from build123d import *

# Parameters (mm, degrees)
F0_R     = 6.35
F1_DEPTH = 2.54
F2_R     = 0.381
F3_DEPTH = 11.938
F4_W     = 0.254
F4_H     = 3.2643415034
F5_DEPTH = 10.7696
F6_R     = 1.524
F7_DEPTH = 2.5654


with BuildPart() as f1:
    # F0 (on Front) → F1 (new body)
    with BuildSketch(Plane.XZ):
        Circle(F0_R)
    extrude(amount=F1_DEPTH)

    # F2 (on Front) → F3 (cut)
    with BuildSketch(Plane.XZ):
        with Locations((0, 2.9252786189)):
            Circle(F2_R)
    extrude(amount=F3_DEPTH, mode=Mode.SUBTRACT)

    # F4 (on Front) → F5 (cut)
    with BuildSketch(Plane.XZ):
        with Locations((-0.0004456008, 4.9322359264)):
            Rectangle(F4_W, F4_H)
    extrude(amount=F5_DEPTH, mode=Mode.SUBTRACT)

    # F6 (on Front) → F7 (join)
    with BuildSketch(Plane.XZ):
        Circle(F6_R)
        with BuildLine():
            add(Edge.make_bspline(
                [(-0.2672408938, -0.7273242873), (-0.3560866168, -0.8291747878), (-0.5301318635, -0.8291747878)],
                knots=[0, 0, 0, 1, 1, 1], degree=2))
            add(Edge.make_bspline(
                [(-0.5301318635, -0.8291747878), (-0.6098620882, -0.8291747878), (-0.6691735969, -0.812402271)],
                knots=[0, 0, 0, 1, 1, 1], degree=2))
            Line((-0.6691735969, -0.812402271), (-0.6691735969, -0.6164798285))
            add(Edge.make_bspline(
                [(-0.6691735969, -0.6164798285), (-0.6084036085, -0.6315507856), (-0.5583291381, -0.6315507856)],
                knots=[0, 0, 0, 1, 1, 1], degree=2))
            add(Edge.make_bspline(
                [(-0.5583291381, -0.6315507856), (-0.4807866329, -0.6315507856), (-0.4473631393, -0.5832994149)],
                knots=[0, 0, 0, 1, 1, 1], degree=2))
            add(Edge.make_bspline(
                [(-0.4473631393, -0.5832994149), (-0.4139396457, -0.5350480441), (-0.4139396457, -0.4324683037)],
                knots=[0, 0, 0, 1, 1, 1], degree=2))
            Line((-0.4139396457, -0.4324683037), (-0.4139396457, 0.6081569771))
            Line((-0.4139396457, 0.6081569771), (-0.1783951708, 0.6081569771))
            Line((-0.1783951708, 0.6081569771), (-0.1783951708, -0.431009824))
            add(Edge.make_bspline(
                [(-0.1783951708, -0.431009824), (-0.1783951708, -0.6254737868), (-0.2672408938, -0.7273242873)],
                knots=[0, 0, 0, 1, 1, 1], degree=2))
        make_face(mode=Mode.SUBTRACT)
        Polygon((0.3328019713, -0.0634729344), (0.3328019713, -0.5024753303), (0.1011467757, -0.5024753303), (0.1011467757, 0.6081569771), (0.7377731738, 0.6081569771), (0.7377731738, 0.415151494), (0.3328019713, 0.415151494), (0.3328019713, 0.1288033088), (0.7095758992, 0.1288033088), (0.7095758992, -0.0634729344), align=None, mode=Mode.SUBTRACT)
    extrude(amount=F7_DEPTH)


solid = f1.part
Could you check a few things on this model? Use its own coordinates, in mm. A direction names the side the tool comes from. Round coordinates to 2 decimals unless told otherwise and drop trailing zeros. Loops run counter-clockwise (first coordinate to the right, second up) from the corner with the lowest first, then second, coordinate; pieces in that order, holes last. Notation, with made-up numbers: (68, 67) -> (81, 67) arc R21 ccw to (81, 104) -> close; hole circle Ø9 at (86, -24.5). An arc over 180 degrees is marked (long way). Use CSV: the item, a comma, the result in double quotes.
(1) For faces 1 (the flat face through (0, -2.565, -1)), 2 (the flat face through (1.3, -2.54, -1.3)), 3 (the flat face through (0.127, -1, 5)), which set-ups out of +Z, -Z, +X, -X, +Y, -Y let a thin tool reach every point of the face, with its end or its side?
Return value:
face 1,"+Z, -Z, +X, -X, -Y"
face 2,"-Y"
face 3,"+Z, +Y, -Y"
(2) Suppose I cut it at A-A on z = 3.75. Write out the boundary of the cut face in (x, y), plus the area to 3 significant figures.
Return value:
outline,"(-5.12, -2.54) -> (-0.13, -2.54) -> (-0.13, 0) -> (-5.12, 0) -> close; (0.13, -2.54) -> (5.12, -2.54) -> (5.12, 0) -> (0.13, 0) -> close"
area,"25.4 mm²"
(3) Suppose I cut it at B-B on y = -0.3. Write out the boundary of the cut face in (x, z), plus the area to 3 significant figures.
Return value:
outline,"(-0.13, 3.3) -> (-0.13, 6.35) arc R6.35 ccw (long way) to (0.13, 6.35) -> (0.13, 3.3) -> (0.07, 3.3) arc R0.38 cw (long way) to (-0.07, 3.3) -> close"
area,"125 mm²"
(4) Will these pins go through, and if not, where does the flat tip stop? pin 1 Ø1.3 at (y, z) = (-1.5, 4.5) entering from -X; pin 2 Ø1 at (x, z) = (-4, 0.5) entering from -Y; pin 3 Ø1.5 at (y, z) = (-0.5, 3) entering from -X.
Return value:
pin 1,"stops at x = -5.05"
pin 2,"stops at y = -2.54"
pin 3,"stops at x = -5.94"
(5) If we mould it in two halves opening along X, with no side actions, what happens to faces 4 (the flat face through (-0.127, -1, 5)), 5 (the flat face through (0, 0, 0))? For each: +X half, -X half, draft (parallel to the pull), parting line (faces both ways), or undercut.
Return value:
face 4,"undercut"
face 5,"draft"
(6) If I drill on probe 1 along Y at (x, z) = (-4.5, 0.25); probe 2 along X at (y, z) = (-0.7, 3.25); probe 3 along X at (y, z) = (-1.6, 4.25), over which ranges is the centre line in solid material (lowest first)? Write a range as [from, to].
Return value:
probe 1,"y = [-2.54, 0]"
probe 2,"x = [-5.46, -0.2], [0.2, 5.46]"
probe 3,"x = [-4.72, -0.13], [0.13, 4.72]"
